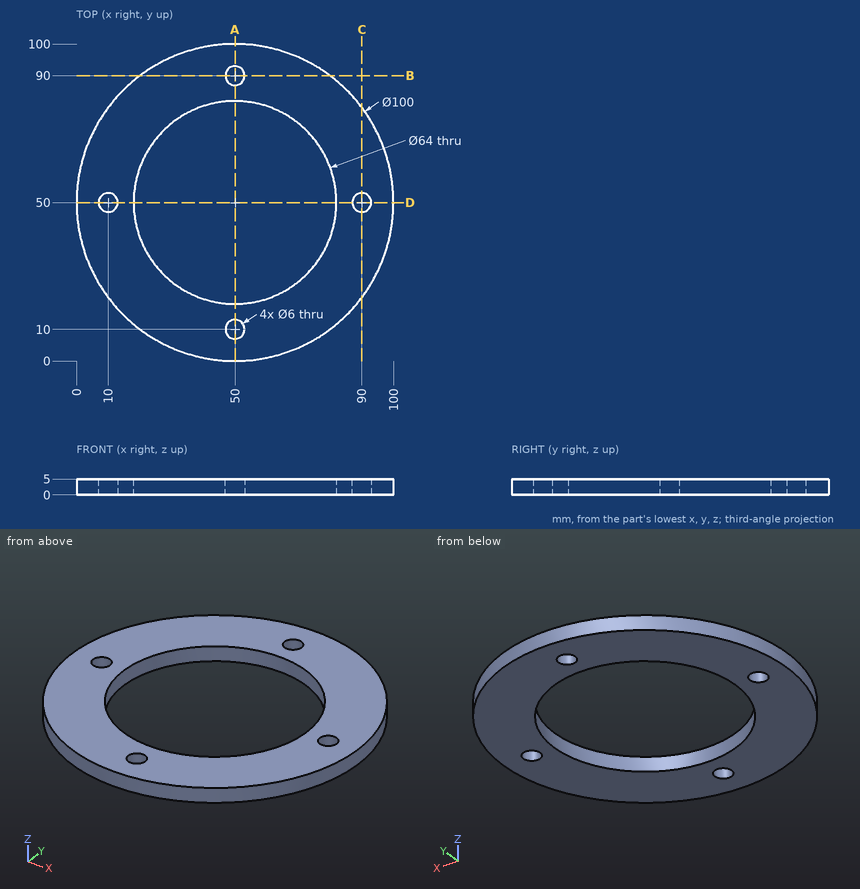
The drawing under review shows one solid part. Ordinate dimensions are in mm from its lowest x, y, z. Coordinates: 2 decimals unless noted, no trailing zeros. Loops run counter-clockwise (first coordinate to the right, second up) from the corner with the lowest first, then second, coordinate; pieces in that order, holes last.
Item 1: Wall thickness on L1, parallel to Y at x = 50, z = 2.6; L2, parallel to Y at x = 41.5, z = 1.35; L3, parallel to Y at x = 87.5, z = 3.5: over which ranges is each line inside the solid? List them lowest first.
Completed:
L1: y = 0 to 7, 13 to 18, 82 to 87, 93 to 100
L2: y = 0.73 to 19.15, 80.85 to 99.27
L3: y = 16.93 to 48.34, 51.66 to 83.07
Item 2: Add section B-B (y = 90). Write out the cut boundary in (x, z).
Completed:
outline: (20, 0) - (47, 0) - (47, 5) - (20, 5) - close; (53, 0) - (80, 0) - (80, 5) - (53, 5) - close
Item 3: Add section A-A (x = 50). Write out the cut boundary in (y, z).
Completed:
outline: (0, 0) - (7, 0) - (7, 5) - (0, 5) - close; (13, 0) - (18, 0) - (18, 5) - (13, 5) - close; (82, 0) - (87, 0) - (87, 5) - (82, 5) - close; (93, 0) - (100, 0) - (100, 5) - (93, 5) - close
Item 4: Clearance check with flat-ended pins moving along their axes: pin 1 (2 mm diameter, centred on y = 52.5, z = 1.5, fed in from -X); pin 2 (3 mm diameter, centred on y = 89, z = 2, fed in from -X); pin 3 (2 mm diameter, centred on y = 10.5, z = 0.5, fed in from -X); pin 4 (5 mm diameter, centred on x = 22.5, y = 41, fed in from +Z). State where each tip first meets the part, or that it passes through.
Completed:
pin 1: stops at x = 0.02
pin 2: stops at x = 16.93
pin 3: stops at x = 18.1
pin 4: passes through
